Model file for the job. Use its own axes, mm. Give positions to 0.01 mm unless a question says otherwise; leave off trailing zeros. Write each loop counter-clockwise with the first axis right and the second up, starting at its lowest first coordinate (ties: lowest second). Pieces come first, ordered by that corner, then holes. Notation, with made-up numbers: (5, 43) - (18, 43) arc R18 cw to (18, 78) - close; hole circle Ø1 at (-27, -26). An arc over 180 degrees is marked (long way). Use a Markdown table: item, result. Add a question column.
Autodesk Inventor part; units mm, degrees
ref_plane "YZ Plane" through (0, 0, 0) normal (1, 0, 0) x (0, 1, 0)
ref_plane "XZ Plane" through (0, 0, 0) normal (0, 1, 0) x (-1, 0, 0)
ref_plane "XY Plane" through (0, 0, 0) normal (0, 0, 1) x (1, 0, 0)
sketch "Sketch1" plane through (0, 0, 0) normal (0, 1, 0) x (-1, 0, 0)
  line L0 (0, 0) -> (150, 0)
  line L1 (150, 0) -> (150, -200)
  line L2 (150, -200) -> (0, -200)
  line L3 (0, -200) -> (0, 0)
  dimension "d0" = 150
  dimension "d1" = 200
extrude "Extrusion1" add sketch "Sketch1" along normal blind 10
sketch "Sketch2" plane through (0, 0, 0) normal (1, 0, 0) x (0, 0, -1)
  line L0 (15, 2.5) -> (185, 2.5)
  line L1 (185, 2.5) -> (185, 7.5)
  line L2 (185, 7.5) -> (15, 7.5)
  line L3 (15, 7.5) -> (15, 2.5)
  point P0 (0, 0)
  dimension "d4" = 170
  dimension "d5" = 5
extrude "Extrusion2" cut sketch "Sketch2" against normal blind 25
properties part number "Chassis Upper - Female"
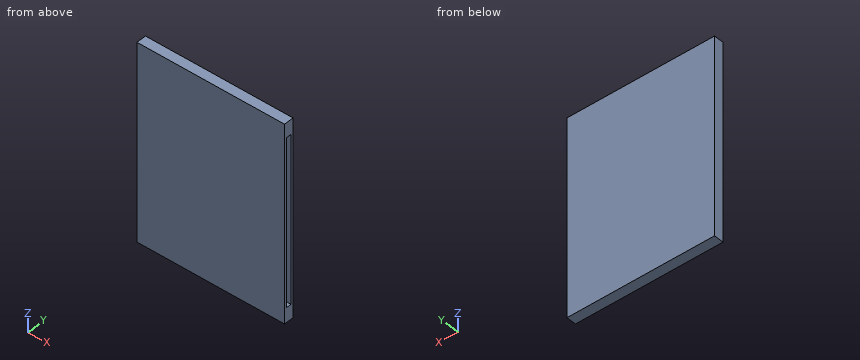
(1) Probe probe 1 along X at (y, z) = (3.75, -27). List the from-to ranges inside material, lowest first. Write a range as [from, to].
(2) Band-saw the part on B-B (z = -22.5). Write the cut outline in (x, y).
(3) Band-saw the part on C-C (y = 5.25). Write the cut outline in (x, z), then the cut area to 4 significant figures.
(4) Band-saw the part on A-A (x = -11). Write the cut outline in (y, z).
(5) Flat gauge pin, fed straight in: pin 1 (4 mm diameter, centred on x = -128, y = 5.5, fed in from +Z). Where does the tip first touch, or does it go through?
Model answer:
| question | item | result |
|---|---|---|
| 1 | probe 1 | x = [-150, -25] |
| 2 | outline | (-150, 0) - (0, 0) - (0, 2.5) - (-25, 2.5) - (-25, 7.5) - (0, 7.5) - (0, 10) - (-150, 10) - close |
| 3 | outline | (-150, -200) - (0, -200) - (0, -185) - (-25, -185) - (-25, -15) - (0, -15) - (0, 0) - (-150, 0) - close |
| 3 | area | 25,750 mm^2 |
| 4 | outline | (0, -200) - (10, -200) - (10, 0) - (0, 0) - close; hole (2.5, -185) - (7.5, -185) - (7.5, -15) - (2.5, -15) - close |
| 5 | pin 1 | stops at z = 0 |
